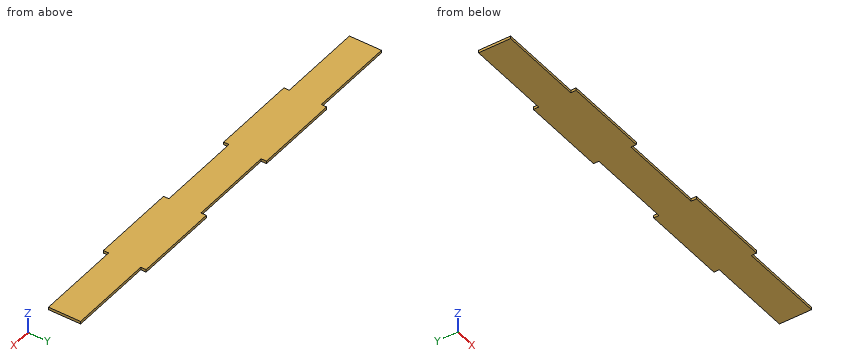
```python
from build123d import *

# Parameters (mm, degrees)
F0_W     = 508
F0_H     = 50.8
F1_DEPTH = 3.175
F2_W     = 101.6
F2_H     = 6.35
F3_DEPTH = 25.4
F4_W     = 101.6
F4_H     = 6.35
F5_DEPTH = 25.4


with BuildPart() as f1:
    # F0 (on Top) → F1 (new body)
    with BuildSketch(Plane.XY):
        with Locations((254, 25.4)):
            Rectangle(F0_W, F0_H)
    extrude(amount=F1_DEPTH)

    # F2 (on face) → F3 (cut)
    with BuildSketch(Plane.XY.offset(3.175)):
        with Locations((254, 3.175)):
            Rectangle(F2_W, F2_H)
        with Locations((457.2, 3.175)):
            Rectangle(F2_W, F2_H)
        with Locations((50.8, 3.175)):
            Rectangle(F2_W, F2_H)
    extrude(amount=-F3_DEPTH, mode=Mode.SUBTRACT)

    # F4 (on face) → F5 (cut)
    with BuildSketch(Plane.XY.offset(3.175)):
        with Locations((457.2, 47.625)):
            Rectangle(F4_W, F4_H)
        with Locations((254, 47.625)):
            Rectangle(F4_W, F4_H)
        with Locations((50.8, 47.625)):
            Rectangle(F4_W, F4_H)
    extrude(amount=-F5_DEPTH, mode=Mode.SUBTRACT)


solid = f1.part
```
Input: part model. Units: mm. Frame: model coordinates. Round coordinates to 2 decimals unless told otherwise and drop trailing zeros. Loops run counter-clockwise (first coordinate to the right, second up) from the corner with the lowest first, then second, coordinate; pieces in that order, holes last. Notation, with made-up numbers: (-7.75, 29.5) -> (40.25, 29.5) arc R14 ccw to (40.25, 40.5) -> close; hole circle Ø1 at (-21.5, 60). An arc over 180 degrees is marked (long way). One line per item, written item: value.
(1) Material intervals for line 1 (X direction, y = 45, z = 1.55); line 2 (Y direction, x = 237, z = 1.3), sorted ascending. Write a range as [from, to].
Geometry check:
line 1: [101.6, 203.2], [304.8, 406.4]
line 2: [6.35, 44.45]
(2) Section A-A (z = 1.6). Return the cut outline in (x, y).
Geometry check:
outline: (0, 6.35) -> (101.6, 6.35) -> (101.6, 0) -> (203.2, 0) -> (203.2, 6.35) -> (304.8, 6.35) -> (304.8, 0) -> (406.4, 0) -> (406.4, 6.35) -> (508, 6.35) -> (508, 44.45) -> (406.4, 44.45) -> (406.4, 50.8) -> (304.8, 50.8) -> (304.8, 44.45) -> (203.2, 44.45) -> (203.2, 50.8) -> (101.6, 50.8) -> (101.6, 44.45) -> (0, 44.45) -> close
(3) Section B-B (x = 438). Return the cut outline in (y, z) (3 decimals), plus the area to 3 significant figures.
Geometry check:
outline: (6.35, 0) -> (44.45, 0) -> (44.45, 3.175) -> (6.35, 3.175) -> close
area: 121 mm2
(4) Pin query (flat end, axial travel): pin 1 (1.6 mm diameter, centred on y = 4.5, z = 1.5, fed in from -X); pin 2 (1.6 mm diameter, centred on x = 72, z = 1.5, fed in from +Y); pin 3 (1 mm diameter, centred on y = 4, z = 1, fed in from +X). Return the tip coordinate at first contact, or that it passes through.
Geometry check:
pin 1: x = 101.6
pin 2: y = 44.45
pin 3: x = 406.4
